Part model, mm, in its own coordinate system. A direction names the side the tool comes from. Coordinates: 2 decimals unless noted, no trailing zeros. Loops run counter-clockwise (first coordinate to the right, second up) from the corner with the lowest first, then second, coordinate; pieces in that order, holes last. Notation, with made-up numbers: M -38.5,-13 L 6.5,-13 A10 ccw 6.5,-3 Z; hole C 49.5,36 d11. An arc over 180 degrees is marked long. Answer as a JSON object with one key per item and string values. Group by question number.
1. Saw through at C-C on x = -41. Write the cut outline in (y, z), then the cut area to 3 significant figures.
2. Drill centre lines: L1, parallel to X at y = 4.75, z = 5.5; L2, parallel to Y at x = -14, z = 13; L3, parallel to X at y = -5.25, z = 6.5. Where is each one in solid material? Low to high.
3. Saw through at A-A on y = 6. Write the cut outline in (x, z).
4. Saw through at D-D on y = -5.25. Write the cut outline in (x, z), then the cut area to 3 significant figures.
5. Mould opens along Y. For faces 1 (the face through (-52.453, 5, 7)), 2 (the face through (51.97, -2.64, 7.6)), 3 (the face through (61, 10.33, 7)) say: released by +Y, released by -Y, zero draft, split by the parting line, or undercut.
6. Drop flat-ended pins along their axis: pin 1 Ø4.5 at (x, z) = (15.5, 5.5) entering from +Y; pin 2 Ø2.5 at (x, z) = (-49.5, 6) entering from -Y; pin 3 Ø1 at (y, z) = (-4, 10) entering from -X; pin 4 Ø3 at (x, y) = (17.5, 1.5) entering from +Z. Give the stop position or say it passes through.
7. 3-axis set-ups, long thin cutter, end or side, ignore diameter. For faces 4 (the face through (-53.85, 9.76, 7.6)), 5 (the face through (61, 8.33, 7)), 6 (the face through (51.37, -7, 7)): which of +Z, -Z, +X, -X, +Y, -Y reach the whole face in a straight line?
from build123d import *

# Parameters (mm, degrees)
F0_W     = 2
F0_H     = 7
F1_DEPTH = 15
F2_R     = 0.99999
F3_R     = 2


# Not quite as in the source:
# - a fillet or chamfer is up to 0.001 mm smaller than in the source, because OpenCascade refuses the exact size


with BuildPart() as f1:
    # F0 (on Top) → F1 (new body)
    with BuildSketch(Plane.XY):
        Polygon((61.5470979531, -0.0695097194), (-52.4529020469, -0.0695097194), (-52.4529020469, -2.0695097194), (49.3698753417, -2.0695097194), (51.3698753417, -2.0695097194), (61.5470979531, -2.0695097194), align=None)
        Polygon((-52.4529020469, -2.0695097194), (-52.4529020469, -0.0695097194), (-52.4529020469, 8.3304902806), (-54.4529020469, 8.3304902806), (-54.4529020469, -2.0695097194), align=None)
        Polygon((61.5470979531, 8.3304902806), (61.5470979531, -0.0695097194), (61.5470979531, -2.0695097194), (63.5470979531, -2.0695097194), (63.5470979531, 8.3304902806), align=None)
        Polygon((-54.4529020469, 8.3304902806), (-52.4529020469, 8.3304902806), (-46.4529020469, 8.3304902806), (-46.4529020469, 10.3304902806), (-54.4529020469, 10.3304902806), align=None)
        Polygon((58.5470979531, 8.3304902806), (61.5470979531, 8.3304902806), (63.5470979531, 8.3304902806), (63.5470979531, 10.3304902806), (58.5470979531, 10.3304902806), align=None)
        with Locations((50.3698753417, -5.5695097194)):
            Rectangle(F0_W, F0_H)
        Polygon((51.3698753417, -9.0695097194), (49.3698753417, -9.0695097194), (41.3698753417, -9.0695097194), (41.3698753417, -11.0695097194), (51.3698753417, -11.0695097194), align=None)
    extrude(amount=F1_DEPTH)

    # F2 (radius 1 in the source; OpenCascade refuses exactly that, so slightly less here)
    f2_edges = [f1.edges().sort_by_distance(p)[0] for p in [
        (58.547098, 10.33049, 7.5),
        (58.547098, 8.33049, 7.5),
        (-46.452902, 8.33049, 7.5),
        (-46.452902, 10.33049, 7.5),
        (41.369875, -9.06951, 7.5),
        (41.369875, -11.06951, 7.5),
    ]]
    fillet(f2_edges, radius=F2_R)

    # F3
    f3_edges = [f1.edges().sort_by_distance(p)[0] for p in [
        (-54.452902, 10.33049, 7.5),
        (-54.452902, -2.06951, 7.5),
        (63.547098, -2.06951, 7.5),
        (63.547098, 10.33049, 7.5),
        (51.369875, -11.06951, 7.5),
        (49.369875, -2.06951, 7.5),
        (51.369875, -2.06951, 7.5),
        (49.369875, -9.06951, 7.5),
        (-52.452902, -0.06951, 7.5),
        (61.547098, -0.06951, 7.5),
    ]]
    fillet(f3_edges, radius=F3_R)


solid = f1.part
Outcome:
{
 "1": {"outline": "M -2.07,0 L -0.07,0 L -0.07,15 L -2.07,15 Z", "area": "30.0 mm²"},
 "2": {"L1": "x = -54.45 to -52.45, 61.55 to 63.55", "L2": "y = -2.07 to -0.07", "L3": "x = 49.37 to 51.37"},
 "3": {"outline": "M -54.45,0 L -52.45,0 L -52.45,15 L -54.45,15 Z; M 61.55,0 L 63.55,0 L 63.55,15 L 61.55,15 Z"},
 "4": {"outline": "M 49.37,0 L 51.37,0 L 51.37,15 L 49.37,15 Z", "area": "30.0 mm²"},
 "5": {"face 1": "undercut", "face 2": "released by -Y", "face 3": "released by +Y"},
 "6": {"pin 1": "stops at y = -0.07", "pin 2": "stops at y = -2.07", "pin 3": "stops at x = 49.29", "pin 4": "passes through"},
 "7": {"face 4": "+Z, -Z, -X, +Y", "face 5": "+Z, -Z", "face 6": "+Z, -Z, +X, -Y"}
}
